Work out the finished part from the listing and answer in its coordinate system (mm). Face numbers are marked on the shaded views. A direction names the side the tool comes from. Round coordinates to 2 decimals unless told otherwise and drop trailing zeros. Write each loop counter-clockwise with the first axis right and the second up, starting at its lowest first coordinate (ties: lowest second). Pieces come first, ordered by that corner, then holes. Notation, with made-up numbers: M 20,-4 L 46,-4 A26 ccw 46,26 Z; hole C 87,26.5 d4. An arc over 180 degrees is marked long. Answer in a Markdown table with one row per item.
```python
from build123d import *

# Parameters (mm, degrees)
BOSS_EXTRUDE1_DEPTH = 21
BOSS_EXTRUDE2_DEPTH = 2
FILLET1_R           = 0.5


with BuildPart() as part:
    # Sketch1 → Boss-Extrude1 (new body)
    with BuildSketch(Plane(origin=(0, 0, 0), x_dir=(1, 0, 0), z_dir=(0, 1, 0))):
        with BuildLine():
            Line((-30, 18.5), (30, 18.5))
            ThreePointArc((30, 18.5), (32.121320344, 17.621320344), (33, 15.5))
            Line((33, 15.5), (33, -15.5))
            ThreePointArc((33, -15.5), (32.121320344, -17.621320344), (30, -18.5))
            Line((30, -18.5), (-30, -18.5))
            ThreePointArc((-30, -18.5), (-32.121320344, -17.621320344), (-33, -15.5))
            Line((-33, -15.5), (-33, 15.5))
            ThreePointArc((-33, 15.5), (-32.121320344, 17.621320344), (-30, 18.5))
        make_face()
        with BuildLine():
            Line((-28, 16.5), (28, 16.5))
            ThreePointArc((28, 16.5), (30.121320344, 15.621320344), (31, 13.5))
            Line((31, 13.5), (31, -13.5))
            ThreePointArc((31, -13.5), (30.121320344, -15.621320344), (28, -16.5))
            Line((28, -16.5), (-28, -16.5))
            ThreePointArc((-28, -16.5), (-30.121320344, -15.621320344), (-31, -13.5))
            Line((-31, -13.5), (-31, 13.5))
            ThreePointArc((-31, 13.5), (-30.121320344, 15.621320344), (-28, 16.5))
        make_face(mode=Mode.SUBTRACT)
    extrude(amount=BOSS_EXTRUDE1_DEPTH)

    # Sketch2 → Boss-Extrude2 (add)
    with BuildSketch(Plane(origin=(0, 21, 0), x_dir=(1, 0, 0), z_dir=(0, 1, 0))):
        with BuildLine():
            Line((-30, 18.5), (30, 18.5))
            ThreePointArc((30, 18.5), (32.121320344, 17.621320344), (33, 15.5))
            Line((33, 15.5), (33, -15.5))
            ThreePointArc((33, -15.5), (32.121320344, -17.621320344), (30, -18.5))
            Line((30, -18.5), (-30, -18.5))
            ThreePointArc((-30, -18.5), (-32.121320344, -17.621320344), (-33, -15.5))
            Line((-33, -15.5), (-33, 15.5))
            ThreePointArc((-33, 15.5), (-32.121320344, 17.621320344), (-30, 18.5))
        make_face()
    extrude(amount=BOSS_EXTRUDE2_DEPTH)

    # Fillet1
    fillet1_edges = [part.edges().sort_by_distance(p)[0] for p in [
        (-32.121320344, 23, 17.621320344),
        (0, 23, 18.5),
        (32.121320344, 23, 17.621320344),
        (33, 23, 0),
        (32.121320344, 23, -17.621320344),
        (0, 23, -18.5),
        (-32.121320344, 23, -17.621320344),
        (-33, 23, 0),
    ]]
    fillet(fillet1_edges, radius=FILLET1_R)


solid = part.part
```
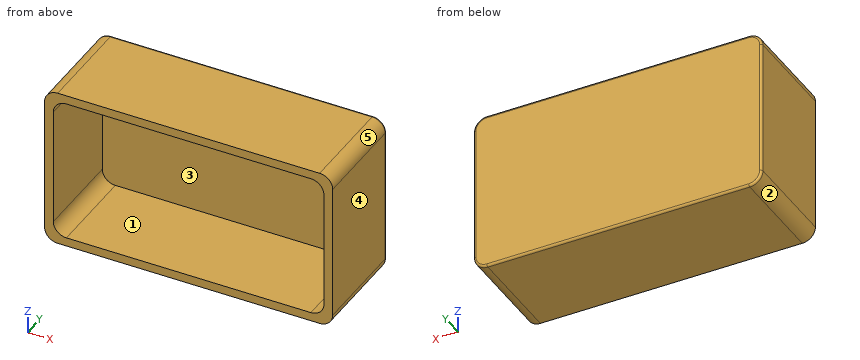
1. A tool of negligible diameter and unlimited length cuts with its end or side. For the marked faces 1 and 2, from which of +Z, -Z, +X, -X, +Y, -Y can it reach the whole face along a straight path? Write none if from no direction.
Calculated:
| item | result |
|---|---|
| face 1 | -Y |
| face 2 | -Z, -X, +Y, -Y |
2. Consider line 1 along Z through (x, y) = (-9.5, 17.75); line 2 along X through (y, z) = (20.5, -3.5); line 3 along Y through (x, z) = (-27, 13.5). Determine where each line is inside the solid, lowest interval first. Write a range as from..to.
Calculated:
| item | result |
|---|---|
| line 1 | z = -18.5..-16.5, 16.5..18.5 |
| line 2 | x = -33..-31, 31..33 |
| line 3 | y = 21..23 |
3. Given pin 1 (2 mm diameter, centred on x = -18, z = 8.5, fed in from -Y), flat-ended and moving along its own axis, determine where the tip first touches the part or whether it passes through.
Calculated:
| item | result |
|---|---|
| pin 1 | stops at y = 21 |
4. The part is cut by section A-A (y = 9.5). Determine the outline of the cut face in (x, z), plus the area to 3 significant figures.
Calculated:
| item | result |
|---|---|
| outline | M -33,-15.5 A3 ccw -30,-18.5 L 30,-18.5 A3 ccw 33,-15.5 L 33,15.5 A3 ccw 30,18.5 L -30,18.5 A3 ccw -33,15.5 Z; hole M -31,-13.5 A3 ccw -28,-16.5 L 28,-16.5 A3 ccw 31,-13.5 L 31,13.5 A3 ccw 28,16.5 L -28,16.5 A3 ccw -31,13.5 Z |
| area | 396 mm² |
5. Determine the mould class of the marked faces 3, 4 and 5 for opening direction Z: released by +Z, released by -Z, zero draft, split by the parting line, or undercut.
Calculated:
| item | result |
|---|---|
| face 3 | undercut |
| face 4 | zero draft |
| face 5 | released by +Z |
6. The part is cut by section B-B (z = -10). Determine the outline of the cut face in (x, y), plus the area to 3 significant figures.
Calculated:
| item | result |
|---|---|
| outline | M -33,0 L -31,0 L -31,21 L 31,21 L 31,0 L 33,0 L 33,22.5 A0.5 ccw 32.5,23 L -32.5,23 A0.5 ccw -33,22.5 Z |
| area | 216 mm² |
7. The part is cut by section C-C (x = -5). Determine the outline of the cut face in (y, z).
Calculated:
| item | result |
|---|---|
| outline | M 0,-18.5 L 22.5,-18.5 A0.5 ccw 23,-18 L 23,18 A0.5 ccw 22.5,18.5 L 0,18.5 L 0,16.5 L 21,16.5 L 21,-16.5 L 0,-16.5 Z |
